Input: part model. Units: mm. Frame: model coordinates. A direction names the side the tool comes from. Give positions to 0.01 mm unless a question says otherwise; leave off trailing zeros. Loops run counter-clockwise (first coordinate to the right, second up) from the corner with the lowest first, then second, coordinate; pieces in that order, holes last. Notation, with made-up numbers: (-36.75, 18) -> (10.25, 18) arc R9 ccw to (10.25, 23) -> close; hole circle Ø8 at (47, -31.5). An arc over 180 degrees is marked (long way). Answer as a JSON object with one key per item and string values. Group by question number.
```python
from build123d import *

# Parameters (mm, degrees)
SKETCH_W             = 410
SKETCH_H             = 61
PAD_DEPTH            = 11.5
SKETCH001_W          = 11
SKETCH001_H          = 3
POCKET_DEPTH         = 410.001
SKETCH002_W          = 5.75
SKETCH002_H          = 5.75
POCKET001_DEPTH      = 410.001
SKETCH003_W          = 3
SKETCH003_H          = 5.75
POCKET002_DEPTH      = 410.001
SKETCH005_W          = 410
SKETCH005_H          = 61
PAD001_DEPTH         = 1
BODY_PLACEMENT_ANGLE = 90


with BuildPart() as part:
    # Sketch → Pad (new body)
    with BuildSketch(Plane.XY):
        with Locations((205, 30.5)):
            Rectangle(SKETCH_W, SKETCH_H)
    extrude(amount=PAD_DEPTH)

    # Sketch001 (on Face4 of Pad) → Pocket (cut, through all)
    with BuildSketch(Plane(origin=(0, 0, 0), x_dir=(0, -1, 0), z_dir=(-1, 0, 0))):
        with Locations((-55.5, 10)):
            Rectangle(SKETCH001_W, SKETCH001_H)
    extrude(amount=-POCKET_DEPTH, mode=Mode.SUBTRACT)

    # Sketch002 (on Face2 of Pocket) → Pocket001 (cut, through all)
    with BuildSketch(Plane(origin=(0, 0, 0), x_dir=(0, -1, 0), z_dir=(-1, 0, 0))):
        with Locations((-6.625, 8.625)):
            Rectangle(SKETCH002_W, SKETCH002_H)
    extrude(amount=-POCKET001_DEPTH, mode=Mode.SUBTRACT)

    # Sketch003 (on Face2 of Pocket001) → Pocket002 (cut, through all)
    with BuildSketch(Plane(origin=(0, 0, 0), x_dir=(0, -1, 0), z_dir=(-1, 0, 0))):
        with Locations((-45.5, 8.625)):
            Rectangle(SKETCH003_W, SKETCH003_H)
    extrude(amount=-POCKET002_DEPTH, mode=Mode.SUBTRACT)

    # Sketch005 (on Face4 of Pocket002) → Pad001 (join)
    with BuildSketch(Plane(origin=(0, 0, 0), x_dir=(1, 0, 0), z_dir=(0, 0, -1))):
        with Locations((205, -30.5)):
            Rectangle(SKETCH005_W, SKETCH005_H)
    extrude(amount=PAD001_DEPTH)


with BuildPart() as part_1:
    # Body placement: moved
    add(part.part.moved(Location((0, 0, -11.5))).rotate(Axis((0, 0, -11.5), (0, 0, 1)), BODY_PLACEMENT_ANGLE))


solid = part_1.part
```
Q1. Section A-A on y = 309.5. Return the cut outline in (x, z).
Q2. Section B-B on x = -54.5. Return the cut outline in (y, z).
Q3. Pull-direction query (Z, two-part tool) for faces 3 (the face through (-30, 202, -12.5)), 4 (the face through (-27, 202, 0)), 5 (the face through (-61, 202, -8)); classes: +Z half, -Z half, draft (parallel to the pull), parting line (faces both ways), or undercut.
Q4. Set-up query: faces 1 (the face through (-56, 202, -3)), 2 (the face through (-31, 0, -6)). Return all of +Z, -Z, +X, -X, +Y, -Y with unobstructed straight access to the full face (end or side cutting, diameter ignored); none if empty.
Q5. Pin query (flat end, axial travel): pin 1 Ø3 at (x, y) = (-7, 175) entering from +Z; pin 2 Ø3.5 at (y, z) = (191.5, -1) entering from -X. Return the tip coordinate at first contact, or that it passes through.
Q6. Ray query, probe 1 along X at (y, z) = (64, -1); probe 2 along X at (y, z) = (276.5, -4); probe 3 along Z at (x, y) = (-57, 109). Return the intervals inside material, ascending.
Numbers:
{
 "1": {"outline": "(-61, -12.5) -> (0, -12.5) -> (0, 0) -> (-3.75, 0) -> (-3.75, -5.75) -> (-9.5, -5.75) -> (-9.5, 0) -> (-44, 0) -> (-44, -5.75) -> (-47, -5.75) -> (-47, 0) -> (-50, 0) -> (-50, -3) -> (-61, -3) -> close"},
 "2": {"outline": "(0, -12.5) -> (410, -12.5) -> (410, -3) -> (0, -3) -> close"},
 "3": {"face 3": "-Z half", "face 4": "+Z half", "face 5": "draft"},
 "4": {"face 1": "+Z, -X, +Y, -Y", "face 2": "+Z, -Z, +X, -X, -Y"},
 "5": {"pin 1": "stops at z = -5.75", "pin 2": "stops at x = -50"},
 "6": {"probe 1": "x = -50 to -47, -44 to -9.5, -3.75 to 0", "probe 2": "x = -61 to -47, -44 to -9.5, -3.75 to 0", "probe 3": "z = -12.5 to -3"}
}
